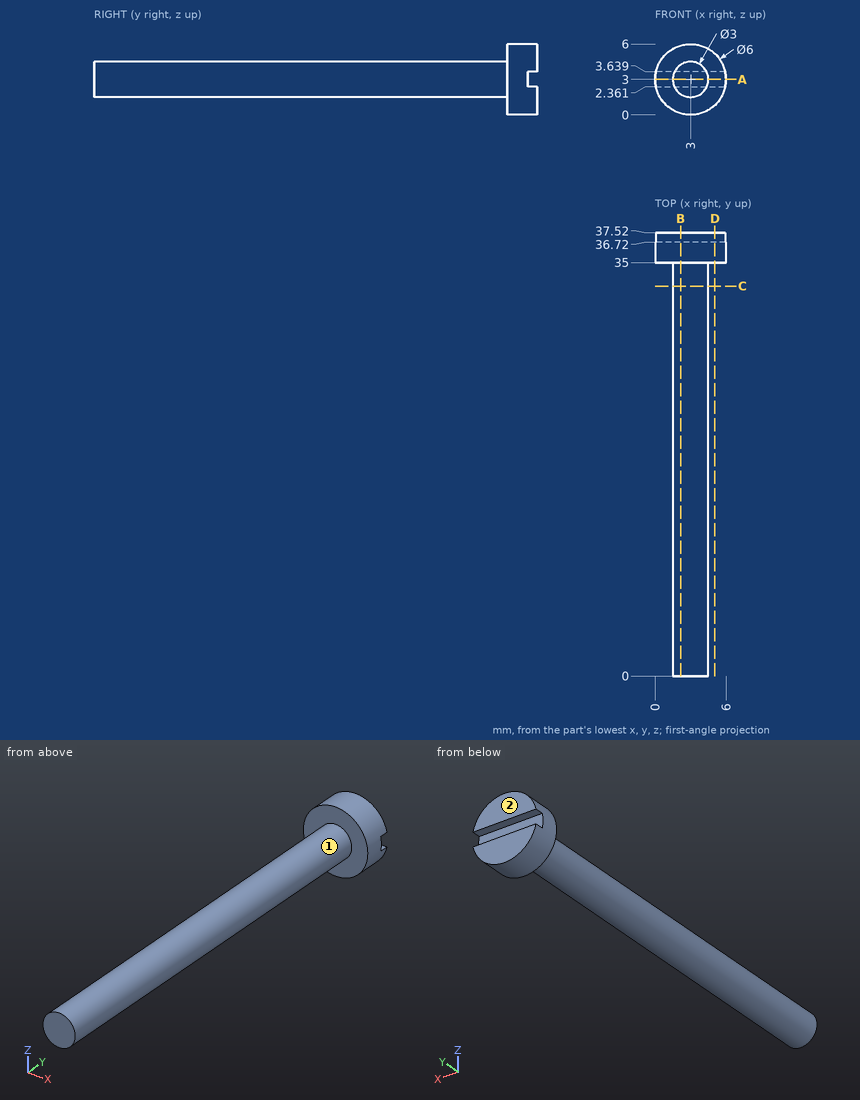
Design review of the part shown in the three views and the two pictorial views. Dimensions are in mm from the part's minimum x, y and z. A direction names the side the tool comes from. Round coordinates to 2 decimals unless told otherwise and drop trailing zeros. Write each loop counter-clockwise with the first axis right and the second up, starting at its lowest first coordinate (ties: lowest second). Pieces come first, ordered by that corner, then holes. Notation, with made-up numbers: (59, 79.5) -> (114, 79.5) arc R13 cw to (114, 92.5) -> close; hole circle Ø9 at (-12, 12.25). An arc over 180 degrees is marked (long way). Answer as a JSON object with one key per item and string values.
1. To check wall thickness, follow line 1 along Y through (x, z) = (1.7, 1.6); line 2 along Y through (x, z) = (2.35, 3.3); line 3 along X through (y, z) = (29, 3.1). State the ranges of each line that lie inside material, in increasing order.
Results found:
{"line 1": "y = 35 to 37.52", "line 2": "y = 0 to 36.72", "line 3": "x = 1.5 to 4.5"}
2. We need section A-A on z = 3. State the section outline as (x, y) points, and give its area (3 significant figures).
Results found:
{"outline": "(0, 35) -> (1.5, 35) -> (1.5, 0) -> (4.5, 0) -> (4.5, 35) -> (6, 35) -> (6, 36.72) -> (0, 36.72) -> close", "area": "115 mm^2"}
3. We need section D-D on x = 5.05. State the section outline as (y, z) points, and give its area (3 significant figures).
Results found:
{"outline": "(35, 0.81) -> (37.52, 0.81) -> (37.52, 2.36) -> (36.72, 2.36) -> (36.72, 3.64) -> (37.52, 3.64) -> (37.52, 5.19) -> (35, 5.19) -> close", "area": "10.0 mm^2"}
4. Machinability: for the marked faces 1 and 2, which of the approach directions +Z, -Z, +X, -X, +Y, -Y give a long, thin tool a straight path to every point of the face, cutting with its end or side? Answer none if there is none.
Results found:
{"face 1": "-Y", "face 2": "+Z, -Z, +X, -X, +Y"}
5. We need section B-B on x = 2.15. State the section outline as (y, z) points.
Results found:
{"outline": "(0, 1.76) -> (35, 1.76) -> (35, 0.12) -> (37.52, 0.12) -> (37.52, 2.36) -> (36.72, 2.36) -> (36.72, 3.64) -> (37.52, 3.64) -> (37.52, 5.88) -> (35, 5.88) -> (35, 4.24) -> (0, 4.24) -> close"}
6. We need section C-C on y = 33. State the section outline as (x, z) points.
Results found:
{"outline": "circle Ø3 at (3, 3)"}
7. Clearance check with flat-ended pins moving along their axes: pin 1 (1.5 mm diameter, centred on y = 17, z = 4.5, fed in from +X); pin 2 (0.6 mm diameter, centred on x = 1.5, y = 37, fed in from -Z); pin 3 (2 mm diameter, centred on y = 27, z = 1, fed in from -X). State where each tip first meets the part, or that it passes through.
Results found:
{"pin 1": "stops at x = 4.3", "pin 2": "stops at z = 0.25", "pin 3": "stops at x = 1.88"}
